Part model, mm, in its own coordinate system. A direction names the side the tool comes from. Round coordinates to 2 decimals unless told otherwise and drop trailing zeros. Loops run counter-clockwise (first coordinate to the right, second up) from the corner with the lowest first, then second, coordinate; pieces in that order, holes last.
from build123d import *

# Parameters (mm, degrees)
FILLET1_R = 3.81
FILLET2_R = 4.572


with BuildPart() as part:
    # Sketch1 → Base-Revolve (revolve)
    with BuildSketch(Plane.XY, mode=Mode.PRIVATE) as base_revolve_sk:
        Polygon((0, 22.698261335), (12.446, 22.698261335), (12.446, 9.490261335), (10.16, 9.490261335), (10.16, 10.760261335), (11.684, 10.760261335), (11.684, 21.428261335), (0, 21.428261335), align=None)
    revolve(base_revolve_sk.sketch.rotate(Axis((0, 0, 0), (0, 1, 0)), 90), axis=Axis((0, 0, 0), (0, 1, 0)))

    # Fillet1
    fillet1_edges = [part.edges().sort_by_distance(p)[0] for p in [
        (0, 21.428261335, 11.684),
    ]]
    fillet(fillet1_edges, radius=FILLET1_R)

    # Fillet2
    fillet2_edges = [part.edges().sort_by_distance(p)[0] for p in [
        (0, 22.698261335, 12.446),
    ]]
    fillet(fillet2_edges, radius=FILLET2_R)


solid = part.part
1) Drop flat-ended pins along their axis: pin 1 Ø2 at (x, y) = (9, 12) entering from -Z; pin 2 Ø4.5 at (x, z) = (-2, -1.5) entering from -Y; pin 3 Ø5 at (y, z) = (19, 7.5) entering from -X; pin 4 Ø8 at (x, z) = (7.5, -0.5) entering from -Y. Give the stop position or say it passes through.
Values:
pin 1: stops at z = -9.53
pin 2: stops at y = 21.43
pin 3: stops at x = -11.36
pin 4: stops at y = 9.49
2) Tool access for faces 5 (the face through (0, 21.428, 0)), 6 (the face through (9.2, 9.49, 4.7)), 7 (the face through (7.11, 14.24, 9.27)): list every direction of +Z, -Z, +X, -X, +Y, -Y with a clear straight run to the whole face (end or side of a thin tool).
Values:
face 5: -Y
face 6: +Z, -Z, +X, -X, -Y
face 7: none
3) Slice it at B-B, the plane y = 16. Give the cut face in (x, z).
Values:
outline: circle Ø24.89 at (0, 0); hole circle Ø23.37 at (0, 0)
4) Slice it at A-A, the plane x = 0. Give the cut face in (y, z), then the cut area to 3 significant figures.
Values:
outline: (9.49, -12.45) - (18.13, -12.45) arc R4.57 ccw to (22.7, -7.87) - (22.7, 7.87) arc R4.57 ccw to (18.13, 12.45) - (9.49, 12.45) - (9.49, 10.16) - (10.76, 10.16) - (10.76, 11.68) - (17.62, 11.68) arc R3.81 cw to (21.43, 7.87) - (21.43, -7.87) arc R3.81 cw to (17.62, -11.68) - (10.76, -11.68) - (10.76, -10.16) - (9.49, -10.16) - close
area: 50.9 mm2
5) Wall check: line 1 along X through (y, z) = (10.1, 0); line 2 along Y through (x, z) = (-5.25, -3.75); line 3 along X through (y, z) = (11.25, -5). Give the ranges that are in metal, low to high.
Values:
line 1: x = -12.45 to -10.16, 10.16 to 12.45
line 2: y = 21.43 to 22.7
line 3: x = -11.4 to -10.56, 10.56 to 11.4
6) Slice it at C-C, the plane z = 0. Give the cut face in (x, y).
Values:
outline: (-12.45, 9.49) - (-10.16, 9.49) - (-10.16, 10.76) - (-11.68, 10.76) - (-11.68, 17.62) arc R3.81 cw to (-7.87, 21.43) - (7.87, 21.43) arc R3.81 cw to (11.68, 17.62) - (11.68, 10.76) - (10.16, 10.76) - (10.16, 9.49) - (12.45, 9.49) - (12.45, 18.13) arc R4.57 ccw to (7.87, 22.7) - (-7.87, 22.7) arc R4.57 ccw to (-12.45, 18.13) - close
7) Mould opens along Z. For faces 1 (the face through (0, 22.698, 0)), 2 (the face through (-10, 10.76, -4)), 3 (the face through (-10.074, 10.134, 1.323)), 4 (the face through (11.042, 13.748, -5.743)) say: released by +Z, released by -Z, zero draft, split by the parting line, or undercut.
Values:
face 1: zero draft
face 2: undercut
face 3: undercut
face 4: split by the parting line
